Could you check a few things on this model? Use its own coordinates, in mm. A direction names the side the tool comes from. Give positions to 0.01 mm unless a question says otherwise; leave off trailing zeros. Loops run counter-clockwise (first coordinate to the right, second up) from the corner with the lowest first, then second, coordinate; pieces in that order, holes last. Notation, with made-up numbers: M -17.75,-20 L 23.25,-20 A31 ccw 23.25,4 Z; hole C 1,-32 d2. An arc over 180 degrees is marked long. Answer in a Markdown table with one row per item. Add a question column.
Autodesk Inventor part; units mm, degrees
ref_plane "Work Plane1" through (30, 0, 0) normal (0, -0.5, 0.8660254) x (1, 0, 0)
ref_plane "YZ Plane" through (0, 0, 0) normal (1, 0, 0) x (0, 1, 0)
ref_plane "XZ Plane" through (0, 0, 0) normal (0, 1, 0) x (-1, 0, 0)
sketch "Sketch1" plane through (0, 0, 0) normal (0, 0, 1) x (1, 0, 0)
  line L0 (-0.0667, 0) -> (8, 0)
  line L1 (8, 0) -> (8, 2)
  line L2 (8, 2) -> (1.4, 2)
  line L3 (1.4, 2) -> (0.9706, 2)
  line L4 (0.9706, 2) -> (0, 2)
  line L5 (0, 2) -> (0, 3.8)
  line L6 (0, 3.8) -> (-2.2, 3.8)
  line L7 (-2.2, 3.8) -> (-2.2, 1.4434)
  line L8 (-2.2, 1.4434) -> (-0.9, 1.4434)
  line L9 (-0.9, 1.4434) -> (-0.0667, 0)
  line L10 (-4.24, 0) -> (10.04, 0)
  line L11 (0, -0.76) -> (0, 4.56)
  line L12 (1.4, 2) -> (0, 2) construction
  dimension "d0" = 6.6
  dimension "d1" = 0.4294
  dimension "d2" = 2.2
  dimension "d3" = 1.3
  dimension "d4" = 60
  dimension "d5" = 4
  dimension "d6" = 4
  dimension "d7" = 2.8868
  dimension "d8" = 7.6
  dimension "d19" = 8
revolve "Body" add sketch "Sketch1" angle 360 about axis through (-0.0667, 0, 0) along (1, 0, 0)
sketch "Sketch2" plane through (-2.2, 0, 0) normal (-1, 0, 0) x (0, 0, 1)
  circle A0 centre (0, 0) radius 1.4434
  line L0 (0, -5.32) -> (0, 5.32)
  line L1 (-5.32, 0) -> (5.32, 0)
  line L2 (1.4434, 0) -> (0.7217, -1.25)
  line L3 (0.7217, -1.25) -> (-0.7217, -1.25)
  line L4 (-0.7217, -1.25) -> (-1.4434, 0)
  line L5 (-1.4434, 0) -> (-0.7217, 1.25)
  line L6 (-0.7217, 1.25) -> (0.7217, 1.25)
  line L7 (0.7217, 1.25) -> (1.4434, 0)
  point P0 (0, 0)
extrude "Slot" add sketch "Sketch2" against normal up to next contours L7 A0 | A0 L2 | L6 L0 A0 | A0 L0 L3 | L0 L6 A0 | A0 L3 L0 | L4 A0 | A0 L5
fillet "Fillet1" radius 1.9 1 edges at (-2.2, -3.8, 0)
thread "Thread"
chamfer "Chamfer1" distance 0.4294 distance2 0.4294 1 edges at (8, -2, 0) measured on face at (8, 0.556, 0.0273)
fillet "Fillet2" radius 0.2 1 edges at (0, -2, 0)
ref_plane "Work Plane1" through (30, 0, 0) normal (0, -0.5, 0.8660254) x (1, 0, 0)
equation "\"d0\" = GEL"
equation "\"d1\" = GAL"
equation "\"d2\" = KOH"
equation "\"d3\" = INTI"
equation "\"d5\" = GD"
equation "\"d6\" = BDM"
equation "\"d7\" = 1.1547 * SW"
equation "\"d8\" = KOD"
equation "\"d19\" = NLG"
equation "\"d16\" = RR"
equation "\"d12\" = GEL"
equation "\"d14\" = -0.5 * SPD + 0.5 * GD"
equation "\"d15\" = GUL"
equation "\"d29\" = R"
equation "\"GD\" = NND"
equation "\"NLG\" = 8"
equation "\"GEL\" = 6.6"
equation "\"KOD\" = 7.6"
equation "\"KOH\" = 2.2"
equation "\"INTI\" = 1.3"
equation "\"GAL\" = 0.61345 * PTC"
equation "\"GUL\" = 0.61345 * PTC"
equation "\"BDM\" = NND"
equation "\"SW\" = 2.5"
equation "\"RR\" = 1.9"
equation "\"SPD\" = 3.14117"
equation "\"d28\" = R"
equation "\"R\" = 0.2"
equation "\"TOA\" = 30deg"
equation "\"THREADDIA\" = 4"
equation "\"KOD1\" = KOD - 2 * RR"
equation "\"PTC\" = 0.7"
equation "\"NND\" = 4"
equation "\"E0\" = 1.155 * SW"
equation "\"GD1\" = THREADDIA - 1.2269 * PTC"
properties part number "ANSI B18.3.4M - M4 x 0.7 x 8, BHSBHCSM" material "Steel, Mild"
Item 1: Suppose I cut it at A-A (x = 1). List the corners of the cut face in (y, z) for me.
Item 2: For P1, Ø3, axis at x = 4.5, y = -0.5, coming from the +Z side; P2, Ø1, axis at x = 4, z = -1.5, coming from the +Y side; P3, Ø2.5, axis at y = 0, z = 2, coming from the +X side; P4, Ø2, axis at x = 5, z = -2.5, coming from the +Y side, each with a flat end and sliding along its axis, tell me the tip position at first contact or that it passes through.
Item 3: I need wall thicknesses on L1, parallel to Y at x = -0.75, z = 0.25; L2, parallel to X at y = -2.5, z = 0.75; L3, parallel to X at y = -0.25, z = -3.25. Which ranges of each line are inside material? Lowest first, please.
Item 4: If we mould it in two halves opening along Z, with no side actions, what happens to faces 4 (the face through (-1.504, -0.616, 1.088)), 5 (the face through (8, 0, 0)), 6 (the face through (-0.12, 0.09, -0.03)), 7 (the face through (4, 0, 2))? For each: +Z half, -Z half, draft (parallel to the pull), parting line (faces both ways), or undercut.
Item 5: For faces 1 (the face through (-0.15, -2.8, -2.57)), 2 (the face through (-1.5, 0.63, 1.08)), 3 (the face through (0, 2, -2)), which set-ups out of +Z, -Z, +X, -X, +Y, -Y let a thin tool reach every point of the face, with its end or its side?
Values found:
| question | item | result |
|---|---|---|
| 1 | outline | C 0,0 d4 |
| 2 | P1 | z = 2 |
| 2 | P2 | y = 1.73 |
| 2 | P3 | x = 8 |
| 2 | P4 | y = 1.32 |
| 3 | L1 | -3.74 to -1.16, 1.16 to 3.74 |
| 3 | L2 | -2.06 to 0 |
| 3 | L3 | -1.63 to 0 |
| 4 | face 4 | undercut |
| 4 | face 5 | draft |
| 4 | face 6 | undercut |
| 4 | face 7 | parting line |
| 5 | face 1 | +X, -X |
| 5 | face 2 | -X |
| 5 | face 3 | +X |
